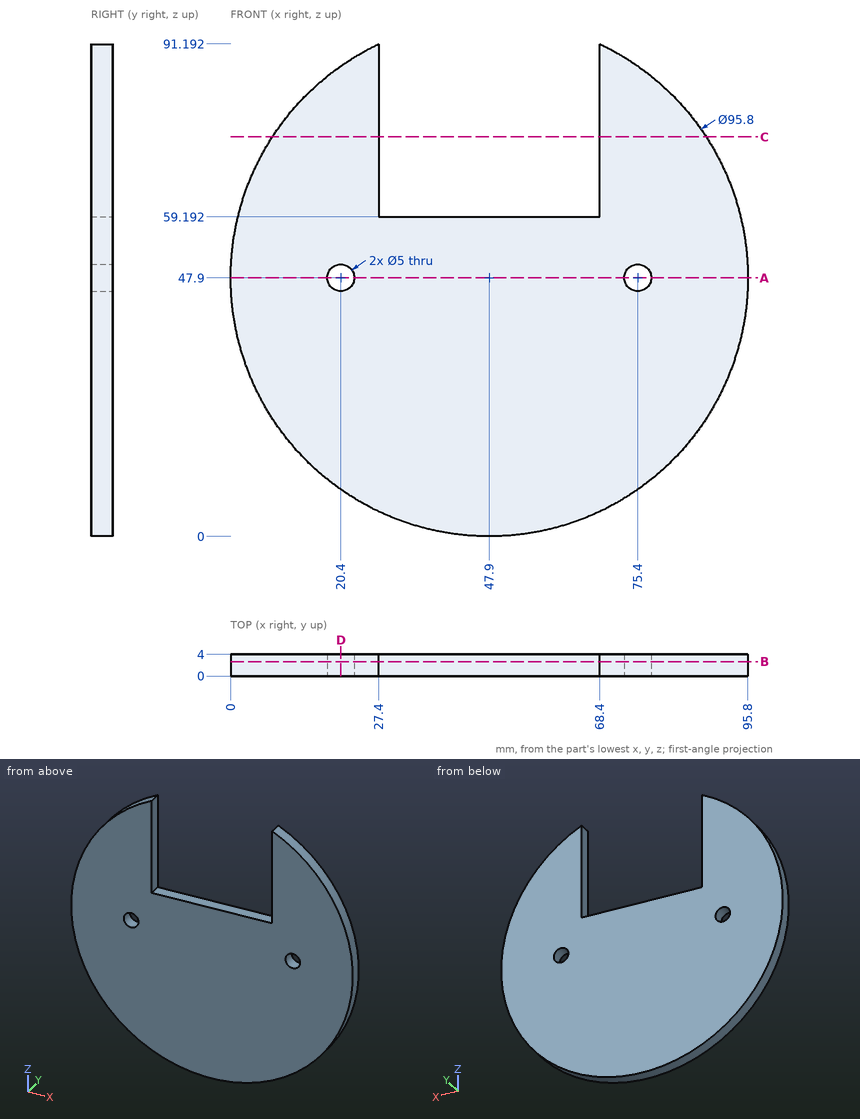
Verification items for this drawing (mm, ordinates from the low corner). Coordinates: 2 decimals unless noted, no trailing zeros. Write each loop counter-clockwise with the first axis right and the second up, starting at its lowest first coordinate (ties: lowest second). Pieces come first, ordered by that corner, then holes. Notation, with made-up numbers: M -30,21 L 5,21 A35 ccw 5,54 Z; hole C 7,-37.75 d4. An arc over 180 degrees is marked long. Use CSV: the item, a comma, the result in double quotes.
Q1. Thickness scan on line 1 along X through (y, z) = (2.85, 47.9); line 2 along X through (y, z) = (3.7, 50) (1 decimal); line 3 along Z through (x, y) = (47.5, 3.25). Record the ranges inside material, lowest first. Write a range as [from, to].
Computed values:
line 1,"[0, 17.9], [22.9, 72.9], [77.9, 95.8]"
line 2,"[0, 19], [21.8, 74], [76.8, 95.8]"
line 3,"[0, 59.19]"
Q2. Section check B-B, the plane y = 2.65. Enter the section's corners in (x, z), and give its area (3 significant figures).
Computed values:
outline,"M 27.4,59.19 L 27.4,91.19 A47.9 ccw long 68.4,91.19 L 68.4,59.19 Z; hole C 20.4,47.9 d5; hole C 75.4,47.9 d5"
area,"5,730 mm²"
Q3. Section check C-C, the plane z = 74. Enter the section's corners in (x, y) (1 decimal), and give its area (3 significant figures).
Computed values:
outline,"M 7.7,0 L 27.4,0 L 27.4,4 L 7.7,4 Z; M 68.4,0 L 88.1,0 L 88.1,4 L 68.4,4 Z"
area,"157 mm²"
Q4. Section check A-A, the plane z = 47.9. Enter the section's corners in (x, y).
Computed values:
outline,"M 0,0 L 17.9,0 L 17.9,4 L 0,4 Z; M 22.9,0 L 72.9,0 L 72.9,4 L 22.9,4 Z; M 77.9,0 L 95.8,0 L 95.8,4 L 77.9,4 Z"
Q5. Go/stop test with flat-tipped pins: P1, Ø1, axis at x = 40.5, y = 1, coming from the +Z side; P2, Ø1.5, axis at y = 2.5, z = 18, coming from the +X side. Record where each tip stops, or that it passes through.
Computed values:
P1,"z = 59.19"
P2,"x = 85.91"
Q6. Section check D-D, the plane x = 20.4. Enter the section's corners in (y, z).
Computed values:
outline,"M 0,8.68 L 4,8.68 L 4,45.4 L 0,45.4 Z; M 0,50.4 L 4,50.4 L 4,87.12 L 0,87.12 Z"
